Part model, mm, in its own coordinate system. A direction names the side the tool comes from. Round coordinates to 2 decimals unless told otherwise and drop trailing zeros. Write each loop counter-clockwise with the first axis right and the second up, starting at its lowest first coordinate (ties: lowest second). Pieces come first, ordered by that corner, then holes. Notation, with made-up numbers: M -21.5,27 L 4.5,27 A24 cw 4.5,47 Z; hole C 19.5,16.5 d4. An arc over 180 degrees is marked long. One line per question, with ' | ' between items. Start each with the question number.
1) Drop flat-ended pins along their axis: pin 1 Ø1.5 at (y, z) = (4, 17.5) entering from +X; pin 2 Ø5 at (x, z) = (8, 5.5) entering from -Y; pin 3 Ø0.9 at (x, y) = (1.5, 11.5) entering from +Z. Give the stop position or say it passes through.
2) Saw through at B-B (y = -22.5). List the corners of the cut face in (x, z).
3) Tool access for faces 4 (the face through (18.752, 0.11, 2.535)), 5 (the face through (-9.99, -0.44, -0.49)), 6 (the face through (0, 11, 8)): list every direction of +Z, -Z, +X, -X, +Y, -Y with a clear straight run to the whole face (end or side of a thin tool).
4) Saw through at A-A (x = 0). Give the number of separate pieces and of enclosed holes in the cut face, plus the area to 3 significant figures.
5) Mould opens along X. For faces 1 (the face through (13.856, -5.745, 22.255)), 2 (the face through (-3, 11, 24)), 3 (the face through (3, -10, 40)) say: pulls with the +X half, pulls with the -X half, needs draft (parallel to the pull), parting line crosses it, or undercut.
6) Saw through at D-D (x = 19.5). List the corners of the cut face in (y, z), plus the area to 3 significant figures.
7) Saw through at C-C (z = 22.5). List the corners of the cut face in (x, y), plus the area to 3 significant figures.
8) Wall check: probe 1 along Y at (x, z) = (0, 1.9); probe 2 along Y at (x, z) = (0, 12); probe 3 along X at (y, z) = (-0.5, 2). Give the ranges that are in metal, low to high. Write a range as [from, to].
```python
from build123d import *

# Parameters (mm, degrees)
CROQUIS1_R              = 27.5
SALIENTE_EXTRUIR1_DEPTH = 5
CROQUIS2_R              = 15
SALIENTE_EXTRUIR2_DEPTH = 35
CROQUIS5_R              = 2.5
CORTAR_EXTRUIR4_DEPTH   = 5
CROQUIS3_R              = 10
CORTAR_EXTRUIR5_DEPTH   = 35
CORTAR_EXTRUIR6_DEPTH   = 32
CROQUIS8_R              = 12.5
CROQUIS8_R_2            = 10
SALIENTE_EXTRUIR4_DEPTH = 1
CROQUIS9_R              = 3
CORTAR_EXTRUIR7_DEPTH   = 25


with BuildPart() as part:
    # Croquis1 → Saliente-Extruir1 (new body)
    with BuildSketch(Plane.XY):
        Circle(CROQUIS1_R)
    extrude(amount=SALIENTE_EXTRUIR1_DEPTH)

    # Croquis2 → Saliente-Extruir2 (add)
    with BuildSketch(Plane.XY.offset(5)):
        Circle(CROQUIS2_R)
    extrude(amount=SALIENTE_EXTRUIR2_DEPTH)

    # Croquis5 → Cortar-Extruir4 (cut)
    with BuildSketch(Plane.XY.offset(5)):
        with Locations((0, 21.25)):
            Circle(CROQUIS5_R)
        with Locations((0, -21.25)):
            Circle(CROQUIS5_R)
        with Locations((21.25, 0)):
            Circle(CROQUIS5_R)
        with Locations((-21.25, 0)):
            Circle(CROQUIS5_R)
        with Locations((15.0260191, 15.0260191)):
            Circle(CROQUIS5_R)
        with Locations((-15.0260191, 15.0260191)):
            Circle(CROQUIS5_R)
        with Locations((-15.0260191, -15.0260191)):
            Circle(CROQUIS5_R)
        with Locations((15.0260191, -15.0260191)):
            Circle(CROQUIS5_R)
    extrude(amount=-CORTAR_EXTRUIR4_DEPTH, mode=Mode.SUBTRACT)

    # Croquis3 → Cortar-Extruir5 (cut)
    with BuildSketch(Plane.XY.offset(40)):
        Circle(CROQUIS3_R)
    extrude(amount=-CORTAR_EXTRUIR5_DEPTH, mode=Mode.SUBTRACT)

    # Croquis7 → Cortar-Extruir6 (cut)
    with BuildSketch(Plane.XY.offset(40)):
        with BuildLine():
            Line((-3, 12.539392014), (-3, 9.539392014))
            ThreePointArc((-3, 9.539392014), (0, 10), (3, 9.539392014))
            Line((3, 9.539392014), (3, 12.539392014))
            Line((3, 12.539392014), (0, 12.539392014))
            Line((0, 12.539392014), (-3, 12.539392014))
        make_face()
    extrude(amount=-CORTAR_EXTRUIR6_DEPTH, mode=Mode.SUBTRACT)

    # Croquis8 → Saliente-Extruir4 (add)
    with BuildSketch(Plane(origin=(0, 0, 0), x_dir=(-1, 0, 0), z_dir=(0, 0, -1))):
        with Locations(Location((0, 0, 0), (0, 0, 180))):
            Circle(CROQUIS8_R)
        with Locations(Location((0, 0, 0), (0, 0, 180))):
            Circle(CROQUIS8_R_2, mode=Mode.SUBTRACT)
    extrude(amount=SALIENTE_EXTRUIR4_DEPTH)

    # Croquis9 → Cortar-Extruir7 (cut, symmetric)
    with BuildSketch(Plane(origin=(0, 0, 0), x_dir=(0, 0, -1), z_dir=(1, 0, 0))):
        with Locations((-22.5, 0)):
            Circle(CROQUIS9_R)
    extrude(amount=CORTAR_EXTRUIR7_DEPTH, both=True, mode=Mode.SUBTRACT)


solid = part.part
```
Answer key:
1) pin 1: stops at x = 14.64 | pin 2: stops at y = -26.93 | pin 3: stops at z = 8
2) outline: M -15.81,0 L -2.17,0 L -2.17,5 L -15.81,5 Z; M 2.17,0 L 15.81,0 L 15.81,5 L 2.17,5 Z
3) face 4: +Z, -Z | face 5: -Z | face 6: +Z
4) separate pieces: 3 | enclosed holes: 0 | area: 499 mm2
5) face 1: parting line crosses it | face 2: undercut | face 3: needs draft
6) outline: M -19.39,0 L -1.79,0 L -1.79,5 L -19.39,5 Z; M 1.79,0 L 19.39,0 L 19.39,5 L 1.79,5 Z | area: 176 mm2
7) outline: M -14.7,-3 A15 ccw 14.7,-3 L 9.54,-3 A10 cw -9.54,-3 Z; M -14.7,3 L -9.54,3 A10 cw -3,9.54 L -3,12.54 L 3,12.54 L 3,9.54 A10 cw 9.54,3 L 14.7,3 A15 ccw Z | area: 316 mm2
8) probe 1: y = [-27.5, -23.75], [-18.75, 18.75], [23.75, 27.5] | probe 2: y = [-15, -10], [12.54, 15] | probe 3: x = [-27.5, -23.7], [-18.8, 18.8], [23.7, 27.5]
